from build123d import *

# Parameters (mm, degrees)
SKETCH1_W                    = 284.5815
SKETCH1_H                    = 30
BASE_FLANGE1_DEPTH           = 2
EDGE_FLANGE1_STRIP_CUT_DEPTH = 30
EDGE_FLANGE1_DEPTH           = 30
EDGE_FLANGE2_STRIP_CUT_DEPTH = 30
EDGE_FLANGE2_DEPTH           = 30
SKETCH10_R                   = 1.5
MOUNTING_HOLES_DEPTH         = 2
SKETCH11_R                   = 1.5
CUT_EXTRUDE2_DEPTH           = 2


# Sheet-metal steps are written as plain solids
with BuildPart() as part:
    # Sketch1 → Base-Flange1 (new body)
    with BuildSketch(Plane(origin=(0, 0, 0), x_dir=(1, 0, 0), z_dir=(0, 1, 0))):
        with Locations((142.29075, -15)):
            Rectangle(SKETCH1_W, SKETCH1_H)
    extrude(amount=-BASE_FLANGE1_DEPTH)

    # Edge-Flange1 strip (across the edge) → Edge-Flange1 strip cut (cut)
    with BuildSketch(Plane(origin=(0, 0, 0), x_dir=(0.9933652782994915, -0.1150018428938158, 0), z_dir=(0, 0, 1))):
        Polygon((-9.511321415, -3.11448322), (1.051314043, -1.891647502), (0.821310357, 0.095083054), (-9.741325101, -1.127752664), align=None)
    extrude(amount=EDGE_FLANGE1_STRIP_CUT_DEPTH, mode=Mode.SUBTRACT)

    # Edge-Flange1 section (across the edge) → Edge-Flange1 (add)
    with BuildSketch(Plane(origin=(0, 0, 0), x_dir=(0.9933652782994915, -0.1150018428938158, 0), z_dir=(0, 0, 1))):
        with BuildLine():
            Line((-2, 0.826795918), (-2, 12.755102041))
            Line((-2, 12.755102041), (0, 12.755102041))
            Line((0, 12.755102041), (0, 0.826795918))
            ThreePointArc((0, 0.826795918), (0.246609229, 0.276806278), (0.821310357, 0.095083054))
            Line((0.821310357, 0.095083054), (1.051314043, -1.891647502))
            ThreePointArc((1.051314043, -1.891647502), (-1.083802855, -1.216513409), (-2, 0.826795918))
        make_face()
    extrude(amount=EDGE_FLANGE1_DEPTH)

    # Edge-Flange2 strip (across the edge) → Edge-Flange2 strip cut (cut)
    with BuildSketch(Plane(origin=(284.5815, 0, 30), x_dir=(-0.9933652782994906, 0.11500184289382274, 0), z_dir=(0, 0, -1))):
        Polygon((-8.988461998, -0.972764326), (0.421885957, -2.062199784), (0.651889643, -0.075469228), (-8.758458312, 1.013966231), align=None)
    extrude(amount=EDGE_FLANGE2_STRIP_CUT_DEPTH, mode=Mode.SUBTRACT)

    # Edge-Flange2 section (across the edge) → Edge-Flange2 (add)
    with BuildSketch(Plane(origin=(284.5815, 0, 30), x_dir=(-0.9933652782994906, 0.11500184289382274, 0), z_dir=(0, 0, -1))):
        with BuildLine():
            Line((-2, 0.656243636), (-2, 13.218181818))
            Line((-2, 13.218181818), (0, 13.218181818))
            Line((0, 13.218181818), (0, 0.656243636))
            ThreePointArc((0, 0.656243636), (0.186610359, 0.166252866), (0.651889643, -0.075469228))
            Line((0.651889643, -0.075469228), (0.421885957, -2.062199784))
            ThreePointArc((0.421885957, -2.062199784), (-1.306709327, -1.164159219), (-2, 0.656243636))
        make_face()
    extrude(amount=EDGE_FLANGE2_DEPTH)

    # Sketch10 → Mounting Holes (cut)
    with BuildSketch(Plane(origin=(-1.986730557, 0.230003686, 0), x_dir=(0, 0, 1), z_dir=(-0.9933652782994914, 0.11500184289381583, 0))):
        with Locations(Location((9, 7.408352498, 0), (0, 0, 270))):
            Circle(SKETCH10_R)
        with Locations(Location((21, 7.408352498, 0), (0, 0, 270))):
            Circle(SKETCH10_R)
    extrude(amount=-MOUNTING_HOLES_DEPTH, mode=Mode.SUBTRACT)

    # Sketch11 → Cut-Extrude2 (cut)
    with BuildSketch(Plane(origin=(282.804519594, -32.740263469, 0), x_dir=(0, 0, -1), z_dir=(0.9933652782994908, -0.11500184289382205, 0))):
        with Locations(Location((-21, 39.945578772, 0), (0, 0, 90))):
            Circle(SKETCH11_R)
        with Locations(Location((-9, 39.945578772, 0), (0, 0, 90))):
            Circle(SKETCH11_R)
    extrude(amount=-CUT_EXTRUDE2_DEPTH, mode=Mode.SUBTRACT)


solid = part.part
Check sheet for the modelled part. Datum: model origin and axes. Units: mm. A direction names the side the tool comes from. Give positions to 0.01 mm unless a question says otherwise; leave off trailing zeros. Loops run counter-clockwise (first coordinate to the right, second up) from the corner with the lowest first, then second, coordinate; pieces in that order, holes last. Notation, with made-up numbers: M 60,-21 L 93,-21 A23 ccw 93,2 Z; hole C 24.5,-31.5 d9. An arc over 180 degrees is marked long. Use a Markdown table: item, result. Add a question column.
Q1. Go/stop test with flat-tipped pins: pin 1 (6 mm diameter, centred on x = 112.5, z = 11.5, fed in from +Y); pin 2 (1 mm diameter, centred on y = 10, z = 6, fed in from +X). Record where each tip stops, or that it passes through.
Q2. Scan lines: line 1 along Y through (x, z) = (37.5, 28.25); line 2 along X through (y, z) = (5, 24); line 3 along X through (y, z) = (3.5, 7.5). Record each from-to range of solid material in increasing order. Write a range as [from, to].
Q3. Sectioned sample at B-B, the plane x = 179. Record the cut outline in (y, z), then the cut area to 3 significant figures.
Q4. Tool access check on faces 1 (the flat face through (285.39, 6.98, 15.21)), 2 (the flat face through (0.79, 6.83, 14.79)), 3 (the flat face through (-1.215, 6.893, 14.79)). Record the directions out of +Z, -Z, +X, -X, +Y, -Y that give a thin tool (end or side, any length) a straight path to the whole face; none if there is none.
Q5. Sectioned sample at A-A, the plane z = 3.75. Record the cut outline in (x, y), then the cut area to 3 significant figures.
Verdict:
| question | item | result |
|---|---|---|
| 1 | pin 1 | y = 0 |
| 1 | pin 2 | x = 287.81 |
| 2 | line 1 | [-2, 0] |
| 2 | line 2 | [-1.43, 0.58], [285.16, 287.17] |
| 2 | line 3 | [-1.61, 0.41], [284.99, 287] |
| 3 | outline | M -2,0 L 0,0 L 0,30 L -2,30 Z |
| 3 | area | 60.0 mm^2 |
| 4 | face 1 | +Z, -Z, +Y |
| 4 | face 2 | +Z, -Z |
| 4 | face 3 | +Z, -Z, -X, +Y |
| 5 | outline | M -1.89,1.05 A2.74 ccw 0.83,-2 L 283.93,-2 A2.74 ccw 286.64,0.42 L 288.09,12.9 L 286.1,13.13 L 284.66,0.65 A0.74 cw 283.93,0 L 0.83,0 A0.74 cw 0.1,0.82 L 1.47,12.67 L -0.52,12.9 Z |
| 5 | area | 626 mm^2 |
